```python
from build123d import *

# Parameters (mm, degrees)
FILLET1_R          = 4.064
SKETCH10_W         = 2.857500069
SKETCH10_H         = 7.5184
REVOLVE3_ANGLE     = 20
CUT_EXTRUDE1_START = 1.27
CUT_EXTRUDE1_DEPTH = 4.9784
CIRPATTERN4_COUNT  = 2
FILLET8_R          = 1.27
FILLET9_R          = 1.27
SKETCH13_W         = 23.8125
SKETCH13_H         = 35.179
SKETCH14_W         = 18.870013955
SKETCH14_H         = 18.870013955
SKETCH14_W_2       = 25.220013955
SKETCH14_H_2       = 25.220013955
CUT_EXTRUDE2_DEPTH = 3.175
SKETCH17_W         = 13.335
SKETCH17_H         = 31.241914403


with BuildPart() as part:
    # Sketch1 → Revolve1 (revolve)
    with BuildSketch(Plane.XY, mode=Mode.PRIVATE) as revolve1_sk:
        Polygon((0, 9.1059), (-20.6375, 9.1059), (-20.6375, 5.042647059), (-17.78, 5.042647059), (-17.78, -5.042647059), (-20.6375, -5.042647059), (-20.6375, -19.7231), (-16.51, -19.7231), (-16.51, -15.5956), (-18.0975, -15.5956), (-18.0975, -13.3096), (-16.51, -13.3096), (-16.51, 6.7564), (-3.8481, 6.7564), (-3.0861, 7.5184), (0, 7.5184), align=None)
    revolve(revolve1_sk.sketch.rotate(Axis((0, 0, 0), (0, 1, 0)), 270), axis=Axis((0, 0, 0), (0, 1, 0)))

    # Fillet1
    # the kernel refuses this fillet: 4.064 mm, written as the material it takes off along each edge
    with BuildSketch(Plane(origin=(0, 9.1059, 0), x_dir=(0, 0, -1), z_dir=(1, 0, 0))) as fillet1_piece_1:
        with BuildLine():
            CenterArc((16.573500069, -4.064), FILLET1_R, 0.010532312, 89.989467688)
            Line((20.6375, -4.063252941), (20.718779999, -4.063238))
            Line((20.718779999, -4.063238), (20.71878, 0))
            Line((20.71878, 0), (20.6375, 0.08128))
            Line((20.6375, 0.08128), (16.573500069, 0.08128))
            Line((16.573500069, 0.08128), (16.573500069, 0))
        make_face()
    revolve(axis=Axis((0, 9.1059, 0), (0, 1, 0)), mode=Mode.SUBTRACT)

    # Sketch10 → Revolve3 (revolve, symmetric)
    with BuildSketch(Plane.XY) as revolve3_sk:
        with Locations((-19.208750034, 0)):
            Rectangle(SKETCH10_W, SKETCH10_H)
    revolve3 = revolve(axis=Axis((0, 0, 0), (0, 1, 0)), revolution_arc=REVOLVE3_ANGLE / 2)
    revolve3 = revolve3 + revolve(revolve3_sk.sketch, axis=Axis((0, 0, 0), (0, -1, 0)), revolution_arc=REVOLVE3_ANGLE / 2)

    # Sketch12 → Cut-Extrude1 (cut)
    with BuildSketch(Plane(origin=(0, -3.7592, 0), x_dir=(1, 0, 0), z_dir=(0, 1, 0)).offset(CUT_EXTRUDE1_START)):
        with BuildLine():
            Line((-7.313638514, 0), (-17.215440903, 1.745954919))
            ThreePointArc((-17.215440903, 1.745954919), (-17.30375, 0), (-17.215440903, -1.745954919))
            Line((-17.215440903, -1.745954919), (-7.313638514, 0))
        make_face()
    cut_extrude1 = extrude(amount=CUT_EXTRUDE1_DEPTH, mode=Mode.SUBTRACT)

    # CirPattern4: Revolve3, Cut-Extrude1 ×2 about axis
    cirpattern4_axis = Axis((0, 0, 0), (0, 1, 0))
    add([revolve3.rotate(cirpattern4_axis, i * 360 / CIRPATTERN4_COUNT) for i in range(1, CIRPATTERN4_COUNT)])
    add([cut_extrude1.rotate(cirpattern4_axis, i * 360 / CIRPATTERN4_COUNT) for i in range(1, CIRPATTERN4_COUNT)], mode=Mode.SUBTRACT)

    # Fillet8
    # the kernel refuses this fillet: 1.27 mm, written as the material it takes off along each edge
    with BuildSketch(Plane(origin=(-16.431533746, -2.4892, -1.607730937), x_dir=(0.1324793231915166, 0, -0.9911857691304479), z_dir=(0, 1, 0)), Plane(origin=(16.431533746, -2.4892, 1.607730937), x_dir=(-0.13247932319151873, 0, 0.9911857691304475), z_dir=(0, 1, 0))) as fillet8_piece_1:
        with BuildLine():
            CenterArc((1.211424462, 1.269207194), FILLET8_R, 201.909884157, 66.065503548)
            Line((0.033154154, 0.795309438), (0.009588748, 0.785831483))
            ThreePointArc((0.009588748, 0.785831483), (-0.008800881, 0.398712653), (-0.025377958, 0.001057934))
            Line((-0.025377958, 0.001057934), (0.000897351, -0.025384144))
            ThreePointArc((0.000897351, -0.025384144), (0.583278445, -0.01509352), (1.165659538, -0.025384144))
            Line((1.165659538, -0.025384144), (1.166556889, 0))
        make_face()
    extrude(amount=4.9784, mode=Mode.SUBTRACT)
    with BuildSketch(Plane(origin=(-16.431533746, -2.4892, 1.607730937), x_dir=(0.13247932319152245, 0, 0.9911857691304472), z_dir=(0, 1, 0)), Plane(origin=(16.431533746, -2.4892, -1.607730937), x_dir=(-0.13247932319151992, 0, -0.9911857691304475), z_dir=(0, 1, 0))) as fillet8_piece_2:
        with BuildLine():
            CenterArc((1.211424462, -1.269207194), FILLET8_R, 92.024612295, 66.065503548)
            Line((0.033154154, -0.795309438), (0.009588748, -0.785831483))
            ThreePointArc((0.009588748, -0.785831483), (-0.008800881, -0.398712653), (-0.025377958, -0.001057934))
            Line((-0.025377958, -0.001057934), (0.000897351, 0.025384144))
            ThreePointArc((0.000897351, 0.025384144), (0.583278445, 0.01509352), (1.165659538, 0.025384144))
            Line((1.165659538, 0.025384144), (1.166556889, 0))
        make_face()
    extrude(amount=4.9784, mode=Mode.SUBTRACT)

    # Fillet9
    fillet9_edges = [part.edges().sort_by_distance(p)[0] for p in [
        (-17.215440903, 0, 1.745954919),
        (-17.215440903, 0, -1.745954919),
        (17.215440903, 0, -1.745954919),
        (17.215440903, 0, 1.745954919),
    ]]
    fillet(fillet9_edges, radius=FILLET9_R)


with BuildPart() as body_2:
    # Sketch13 → Revolve4 (revolve)
    with BuildSketch(Plane.XY):
        with Locations((-11.90625, -5.3086)):
            Rectangle(SKETCH13_W, SKETCH13_H)
    revolve(axis=Axis((0, 12.2809, 0), (0, -1, 0)))

    # Intersect1: read off the stored shape, not the designer's step
    # Intersect1: cut part
    add(part.part, mode=Mode.SUBTRACT)

    # Sketch14 → Cut-Extrude2 (cut)
    with BuildSketch(Plane.XZ.offset(22.8981)):
        with Locations((-18.960006978, 18.960006978)):
            Rectangle(SKETCH14_W, SKETCH14_H)
        with Locations((15.785006978, 18.960006978)):
            Rectangle(SKETCH14_W_2, SKETCH14_H)
        with Locations((-18.960006978, -15.785006978)):
            Rectangle(SKETCH14_W, SKETCH14_H_2)
        with Locations((18.960006978, -18.960006978)):
            Rectangle(SKETCH14_W, SKETCH14_H)
    extrude(amount=-CUT_EXTRUDE2_DEPTH, mode=Mode.SUBTRACT)

    # Sketch16 → Cut-Revolve4 (revolve, cut)
    with BuildSketch(Plane.XY):
        Polygon((17.616090936, -19.7231), (24.456472079, -19.7231), (24.456472079, 14.393066261), (0, 14.393066261), (0, 7.5184), (17.616090936, 7.5184), (17.616090936, -12.224103068), (18.894097, -12.224103068), (18.894097, -16.204339712), (17.616090936, -16.204339712), align=None)
    revolve(axis=Axis((0, 0, 0), (0, -1, 0)), mode=Mode.SUBTRACT)

    # Sketch17 → Cut-Revolve5 (revolve, cut)
    with BuildSketch(Plane.XY, mode=Mode.PRIVATE) as cut_revolve5_sk:
        with Locations((6.6675, -12.039557201)):
            Rectangle(SKETCH17_W, SKETCH17_H)
    revolve(cut_revolve5_sk.sketch.rotate(Axis((0, 3.5814, 0), (0, -1, 0)), 180), axis=Axis((0, 3.5814, 0), (0, -1, 0)), mode=Mode.SUBTRACT)


solid = body_2.part
```
Work out the finished part from the listing and answer in its coordinate system (mm). A direction names the side the tool comes from. Round coordinates to 2 decimals unless told otherwise and drop trailing zeros. Loops run counter-clockwise (first coordinate to the right, second up) from the corner with the lowest first, then second, coordinate; pieces in that order, holes last. Notation, with made-up numbers: (26.25, 69.5) -> (48.25, 69.5) arc R8 ccw to (48.25, 79.5) -> close; hole circle Ø2 at (10, 36.25). An arc over 180 degrees is marked (long way). Write each question's results on one line, items separated by ' | '. Start each with the question number.
1. Given pin 1 Ø2 at (y, z) = (-3, 12.5) entering from +X; pin 2 Ø13.5 at (x, z) = (0.5, 2) entering from -Y; pin 3 Ø11.5 at (x, z) = (-2, 16.5) entering from +Y; pin 4 Ø4.5 at (x, z) = (11, -11) entering from -Y, each flat-ended and moving along its own axis, determine where each tip first touches the part or whether it passes through.
2. A tool of negligible diameter and unlimited length cuts with its end or side. For faces 4 (the face through (11, -19.723, -11)), 5 (the face through (-18, -21, -3.175)), 6 (the face through (-11, -19.723, 11)), 7 (the face through (-0.137, -21.288, -23.812)), 8 (the face through (-3.207, -21.288, 23.596)), from which of +Z, -Z, +X, -X, +Y, -Y can it reach the whole face along a straight path? Write none if from no direction.
3. Section D-D (y = -3.5) is taken. Determine the outline of the cut face in (x, z) (3 decimals), plus the area to 3 significant figures.
4. Section C-C (y = -15) is taken. Determine the outline of the cut face in (x, z) (1 decimal).
5. Find the intervals of material crossed by probe 1 along Y at (x, z) = (6, -19); probe 2 along Y at (x, z) = (11.5, -12); probe 3 along X at (y, z) = (-13, 5.5), in increasing order. Write a range as from..to.
6. Section B-B (x = 0) is taken. Determine the outline of the cut face in (y, z) (1 decimal), plus the area to 3 significant figures.
7. For a pull along Y with two mould halves and no side action, classify faces 1 (the face through (0, 3.581, 0)), 2 (the face through (10.05, -17.63, 13.1)), 3 (the face through (9.525, -21, -16)) as +Y half, -Y half, draft (parallel to the pull), parting line (faces both ways), or undercut.
Evaluation:
1) pin 1: stops at x = 11.85 | pin 2: stops at y = 3.58 | pin 3: stops at y = 6.76 | pin 4: stops at y = -22.9
2) face 4: -Z, +X, -Y | face 5: -Z, -X, -Y | face 6: +Z, -X, -Y | face 7: -Z, +Y, -Y | face 8: +Z, +Y, -Y
3) outline: circle Ø33.02 at (0, 0); hole circle Ø26.67 at (0, 0) | area: 298 mm2
4) outline: circle Ø36.2 at (0, 0); hole circle Ø26.7 at (0, 0)
5) probe 1: y = -22.9..-19.72 | probe 2: y = -15.6..-13.31 | probe 3: x = -15.57..-12.15, 12.15..15.57
6) outline: (-22.9, -23.8) -> (-19.7, -23.8) -> (-19.7, -16.5) -> (-15.6, -16.5) -> (-15.6, -18.1) -> (-13.3, -18.1) -> (-13.3, -16.5) -> (6.8, -16.5) -> (6.8, -3.8) -> (7.5, -3.1) -> (7.5, 3.1) -> (6.8, 3.8) -> (6.8, 16.5) -> (-13.3, 16.5) -> (-13.3, 18.1) -> (-15.6, 18.1) -> (-15.6, 16.5) -> (-19.7, 16.5) -> (-19.7, 23.8) -> (-22.9, 23.8) -> (-22.9, 13.3) -> (3.6, 13.3) -> (3.6, -13.3) -> (-22.9, -13.3) -> close | area: 332 mm2
7) face 1: -Y half | face 2: undercut | face 3: draft
